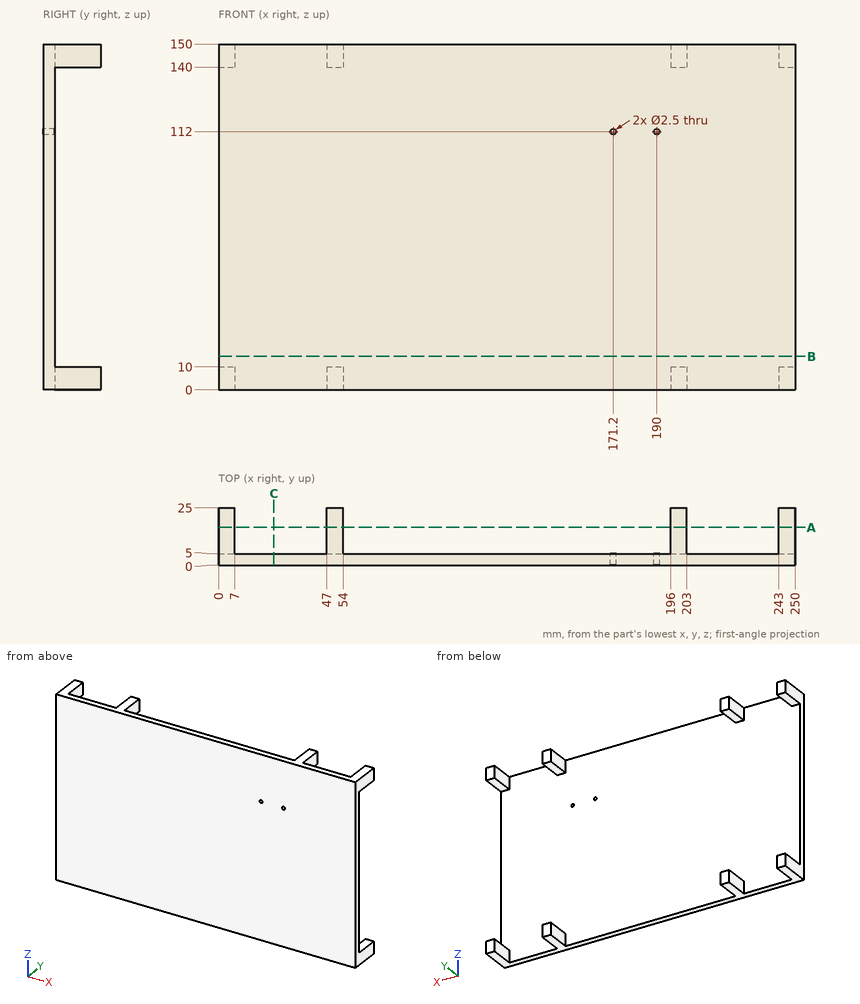
Geometry: see drawing. Coordinates: mm, zero at the bounding-box minimum. Round coordinates to 2 decimals unless told otherwise and drop trailing zeros. Write each loop counter-clockwise with the first axis right and the second up, starting at its lowest first coordinate (ties: lowest second). Pieces come first, ordered by that corner, then holes. Notation, with made-up numbers: (-13.5, 74.25) -> (6.5, 74.25) arc R23 ccw to (6.5, 89.25) -> close; hole circle Ø9 at (-2.75, 89). An arc over 180 degrees is marked (long way). Answer as CSV lines item,"result".
1. Contact query for flat-ended pins moving along their axis: P1, Ø2, axis at x = 146, z = 95, coming from the -Y side; P2, Ø1.5, axis at x = 190, z = 112, coming from the +Y side; P3, Ø1, axis at x = 99.5, z = 75.5, coming from the +Y side. Output: stop coordinate, or through.
Geometry says:
P1,"stops at y = 0"
P2,"passes through"
P3,"stops at y = 5"
2. Section C-C (x = 24). Return the cut outline in (y, z), plus the area to 3 significant figures.
Geometry says:
outline,"(0, 0) -> (5, 0) -> (5, 150) -> (0, 150) -> close"
area,"750 mm^2"
3. Ray query, L1, parallel to X at y = 3.6, z = 112; L2, parallel to Z at x = 190, y = 2; L3, parallel to Y at x = 51, z = 31. Return the intervals inside material, ascending. Write a range as [from, to].
Geometry says:
L1,"x = [0, 169.95], [172.45, 188.75], [191.25, 250]"
L2,"z = [0, 110.75], [113.25, 150]"
L3,"y = [0, 5]"
4. Section A-A (y = 16.5). Give the number of separate pieces and of enclosed holes in the cut face, plus the area to 3 significant figures.
Geometry says:
separate pieces,"8"
enclosed holes,"0"
area,"560 mm^2"
5. Section B-B (z = 14.5). Return the cut outline in (x, y).
Geometry says:
outline,"(0, 0) -> (250, 0) -> (250, 5) -> (0, 5) -> close"
